Autodesk Inventor part; units mm, degrees
ref_plane "YZ Plane" through (0, 0, 0) normal (1, 0, 0) x (0, 1, 0)
ref_plane "XZ Plane" through (0, 0, 0) normal (0, 1, 0) x (-1, 0, 0)
ref_plane "XY Plane" through (0, 0, 0) normal (0, 0, 1) x (1, 0, 0)
sketch "Sketch1" plane through (0, 0, 0) normal (1, 0, 0) x (0, 1, 0)
  line L0 (0, 0) -> (40, 0) construction
  line L1 (40, 0) -> (40, 66.5) construction
  line L2 (40, 66.5) -> (0, 66.5) construction
  line L3 (0, 66.5) -> (0, 0) construction
  line L4 (0, 66.5) -> (40, 66.5) construction
  line L5 (40, 66.5) -> (40, 86.5) construction
  line L6 (40, 86.5) -> (0, 86.5)
  line L7 (0, 86.5) -> (0, 66.5) construction
  line L8 (0, 0) -> (40, 0) construction
  line L9 (40, 0) -> (40, -20) construction
  line L10 (40, -20) -> (0, -20) construction
  line L11 (0, -20) -> (0, 0) construction
  line L12 (48.2, 61.45) -> (-8.2, 61.45) construction
  line L13 (-8.2, 61.45) -> (-8.2, 5.05) construction
  line L14 (-8.2, 5.05) -> (48.2, 5.05) construction
  line L15 (48.2, 5.05) -> (48.2, 61.45) construction
  line L16 (48.2, 33.25) -> (-8.2, 33.25) construction
  line L17 (40, 33.25) -> (0, 33.25) construction
  line L18 (43.57, 56.82) -> (-3.57, 56.82) construction
  line L19 (-3.57, 56.82) -> (-3.57, 9.68) construction
  line L20 (-3.57, 9.68) -> (43.57, 9.68) construction
  line L21 (43.57, 9.68) -> (43.57, 56.82) construction
  line L22 (43.57, 56.82) -> (48.2, 56.82) construction
  line L23 (43.57, 56.82) -> (43.57, 61.45) construction
  line L24 (-3.57, 9.68) -> (-8.2, 9.68) construction
  line L25 (-3.57, 9.68) -> (-3.57, 5.05) construction
  line L26 (40, -10) -> (0, -10) construction
  line L27 (40, 76.5) -> (0, 76.5) construction
  circle A0 centre (30, 76.5) radius 2.1
  circle A1 centre (10, 76.5) radius 2.1
  circle A2 centre (30, -10) radius 2.1
  circle A3 centre (10, -10) radius 2.1
  circle A4 centre (43.57, 56.82) radius 2.6 construction
  circle A5 centre (43.57, 9.68) radius 2.6 construction
  circle A6 centre (-3.57, 9.68) radius 2.6 construction
  circle A7 centre (-3.57, 56.82) radius 2.6 construction
  circle A8 centre (-25, 18.25) radius 11.08 construction
  circle A9 centre (-25, 18.25) radius 13 construction
  circle A10 centre (-25, 18.25) radius 2.5
  line L28 (-60, 153.25) -> (-60, -86.75) construction
  circle A11 centre (-60, -86.75) radius 2.6
  circle A12 centre (-60, 153.25) radius 2.6
  line L29 (-120.2, 153.25) -> (-120.2, -86.75) construction
  circle A13 centre (-120.2, -86.75) radius 2.6
  circle A14 centre (-120.2, 153.25) radius 2.6
  circle A15 centre (-60, -86.75) radius 12 construction
  circle A16 centre (-120.2, -86.75) radius 12 construction
  circle A17 centre (-120.2, 153.25) radius 12 construction
  circle A18 centre (-60, 153.25) radius 12 construction
  line L30 (-110, 482.7599) -> (-70, 482.7599) construction
  line L31 (-70, -517.2401) -> (-110, -517.2401) construction
  circle A19 centre (-25, 48.25) radius 2.5
  circle A20 centre (-25, 48.25) radius 11.08 construction
  circle A21 centre (-25, 48.25) radius 13 construction
  circle A22 centre (20, 33.25) radius 11.08 construction
  circle A23 centre (20, 33.25) radius 13 construction
  line L32 (-23.1873, 29.1807) -> (18.1873, 22.3193) construction
  line L33 (18.1873, 44.1807) -> (-23.1873, 37.3193) construction
  line L34 (-120.8333, -99.25) -> (-47.8333, -99.25)
  line L35 (-47.8333, 165.75) -> (-120.8333, 165.75)
  line L36 (-132.8333, 153.75) -> (-132.8333, -87.25)
  line L37 (-60, 153.25) -> (-120.2, 153.25) construction
  line L38 (-120.2, -86.75) -> (-60, -86.75) construction
  line L39 (-60, 153.25) -> (-60, 165.75) construction
  line L40 (-120.2, -86.75) -> (-120.2, -99.25) construction
  line L41 (48.3276, -20) -> (48.3276, 86.5)
  line L42 (17.6122, 86.5) -> (40, 86.5) construction
  arc A24 (-120.8333, 165.75) -> (-132.8333, 153.75) centre (-120.8333, 153.75) ccw
  arc A25 (-132.8333, -87.25) -> (-120.8333, -99.25) centre (-120.8333, -87.25) ccw
  line L43 (48.3276, -20) -> (-47.8333, -99.25)
  line L44 (-47.8333, 165.75) -> (-47.8333, -99.25) construction
  line L45 (-120.2, -86.75) -> (-132.8333, -86.75) construction
  line L46 (-60, 153.25) -> (-47.8333, 153.25) construction
  line L47 (-36.08, 48.25) -> (-36.08, 286.613) construction
  line L48 (-47.8333, 145.75) -> (-47.8333, 86.5)
  line L49 (-47.8333, 86.5) -> (16.8804, 86.5)
  line L50 (-47.8333, -73.3332) -> (16.8804, -20)
  line L51 (-47.8333, -20) -> (16.8804, -20)
  line L52 (-47.8333, -73.3332) -> (-47.8333, -20)
  line L53 (48.3276, 86.5) -> (48.3276, 165.75)
  line L54 (48.3276, 165.75) -> (-47.8333, 165.75)
  line L55 (-47.8333, 145.75) -> (28.3276, 145.75)
  line L56 (28.3276, 145.75) -> (28.3276, 86.5)
  line L57 (-47.8333, 145.75) -> (28.3276, 86.5) construction
  line L58 (-39.6904, 145.75) -> (28.3276, 92.8349)
  line L59 (-47.8333, 139.4151) -> (20.1847, 86.5)
  circle A26 centre (20, 33.25) radius 3.5
  line L60 (20, 33.25) -> (20, 13.25) construction
  line L61 (20, 33.25) -> (20, 53.25) construction
  circle A27 centre (20, 13.25) radius 2.6
  circle A28 centre (20, 53.25) radius 2.6
  point P0 (-132.8333, -99.25)
  point P1 (-132.8333, 165.75)
  point P2 (-47.8333, 139.8332)
  point P3 (0, 86.5)
  point P4 (0, 86.5)
  dimension "d181" = 22.16
  dimension "d156" = 40
  dimension "d157" = 66.5
  dimension "d158" = 40
  dimension "d159" = 20
  dimension "d160" = 40
  dimension "d161" = 20
  dimension "d162" = 56.4
  dimension "d163" = 56.4
  dimension "d164" = 0
  dimension "d165" = 8.2
  dimension "d166" = 47.14
  dimension "d167" = 47.14
  dimension "d168" = 4.2
  dimension "d169" = 20
  dimension "d170" = 10
  dimension "d171" = 10
  dimension "d172" = 20
  dimension "d173" = 4.2
  dimension "d174" = 4.2
  dimension "d175" = 4.2
  dimension "d176" = 5.2
  dimension "d177" = 5.2
  dimension "d178" = 5.2
  dimension "d179" = 5.2
  dimension "d182" = 26
  dimension "d183" = 5
  dimension "d184" = 240
  dimension "d185" = 60
  dimension "d186" = 5.2
  dimension "d187" = 5.2
  dimension "d188" = 5.2
  dimension "d189" = 5.2
  dimension "d190" = 60.2
  dimension "d191" = 24
  dimension "d192" = 24
  dimension "d193" = 24
  dimension "d194" = 24
  dimension "d195" = 40
  dimension "d196" = 1000
  dimension "d198" = 5
  dimension "d199" = 22.16
  dimension "d200" = 26
  dimension "d202" = 22.16
  dimension "d203" = 26
  dimension "d205" = 15
  dimension "d206" = 265
  dimension "d207" = 85
  dimension "d208" = 106.5
  dimension "d209" = 12
  dimension "d210" = 72.8333
  dimension "d212" = 53.25
  dimension "d213" = 85
  dimension "d214" = 132.5
  dimension "d215" = 60.2
  dimension "d216" = 20
  dimension "d217" = 20
  dimension "d218" = 5
  dimension "d219" = 5
  dimension "d220" = 7
  dimension "d221" = 20
  dimension "d222" = 20
  dimension "d223" = 5.2
  dimension "d224" = 5.2
extrude "Extrusion1" add sketch "Sketch1" along normal blind 3.175 contours L6 L59 L48 L55 L58 L56 | A25 L36 A24 L35 L54 L53 L41 L43 L34
sketch "Sketch4" plane through (3.175, 0, 0) normal (1, 0, 0) x (0, 0, -1)
  line L0 (20, 16.8804) -> (73.3332, -47.8333)
  line L1 (39.0796, -6.2705) -> (54.5136, 6.4492) construction
  line L2 (99.25, -47.8333) -> (20, 48.3276) construction
  line L3 (46.7966, 0.0893) -> (37.2568, 11.6648) construction
  line L4 (46.7966, 0.0893) -> (56.3364, -11.4861) construction
  circle A0 centre (37.2568, 11.6648) radius 2.6
  circle A1 centre (56.3364, -11.4861) radius 2.6
  line L5 (-145.75, 28.3276) -> (-92.8349, 28.3276)
  line L6 (-119.2924, 28.3276) -> (-119.2924, 48.3276) construction
  line L7 (20, 48.3276) -> (-165.75, 48.3276) construction
  line L8 (-119.2924, 38.3276) -> (-104.2924, 38.3276) construction
  line L9 (-119.2924, 38.3276) -> (-134.2924, 38.3276) construction
  circle A2 centre (-134.2924, 38.3276) radius 2.6
  circle A3 centre (-104.2924, 38.3276) radius 2.6
  point P0 (0, 0)
  point P1 (0, 0)
  dimension "d228" = 30
  dimension "d229" = 15
  dimension "d230" = 15
  dimension "d231" = 5.2
  dimension "d232" = 5.2
  dimension "d233" = 15
  dimension "d234" = 15
  dimension "d235" = 5.2
  dimension "d236" = 5.2
  dimension "d237" = 52.9151
  dimension "d238" = 26.4576
extrude "Extrusion4" cut sketch "Sketch4" against normal through all
fillet "Fillet2" radius 3.175 11 edges at (1.5875, 28.3276, 92.8349) (1.5875, 20.1847, 86.5) (1.5875, -39.6904, 145.75) (1.5875, -47.8333, 139.4151) (1.5875, 16.8804, -20) (1.5875, 48.3276, -20) (1.5875, -47.8333, -20) (1.5875, -47.8333, -73.3332) (1.5875, -47.8333, -99.25) (1.5875, -47.8333, 86.5) (1.5875, 28.3276, 145.75)
chamfer "Chamfer1" distance 10 angle 45 1 edges at (1.5875, 48.3276, 165.75)
sketch "Sketch5" plane through (3.175, 0, 0) normal (1, 0, 0) x (0, 0, -1)
  line L0 (-145.75, -30.4384) -> (-145.75, 25.1526)
  line L1 (-165.75, 38.3276) -> (-165.75, -120.8333)
  line L2 (-145.75, 28.3276) -> (-165.75, 28.3276)
  line L3 (-165.75, 28.3276) -> (-165.75, -21.6724)
  line L4 (-165.75, -21.6724) -> (-145.75, -21.6724)
  line L5 (-145.75, -21.6724) -> (-145.75, 28.3276)
  line L6 (18.5023, 48.3276) -> (-155.75, 48.3276)
  line L7 (-142.575, 28.3276) -> (-99.3275, 28.3276)
  line L8 (-155.75, 28.3276) -> (-155.75, -21.6724) construction
  circle A0 centre (-155.75, 15.8276) radius 2.6
  circle A1 centre (-155.75, -9.1724) radius 2.6
  point P0 (0, 0)
  dimension "d239" = 50
  dimension "d241" = 5.2
  dimension "d242" = 5.2
  dimension "d243" = 12.5
  dimension "d244" = 12.5
extrude "Extrusion5" cut sketch "Sketch5" against normal up to next contours A0 | A1
properties part number "X Axis V Wheel Frame Machined"
Verification items for the finished model (mm, model axes). A direction names the side the tool comes from. Give positions to 0.01 mm unless a question says otherwise; leave off trailing zeros. Loops run counter-clockwise (first coordinate to the right, second up) from the corner with the lowest first, then second, coordinate; pieces in that order, holes last.
1. Section check A-A, the plane z = 33.25. Enter the section's corners in (x, y) (3 decimals).
2. Thickness scan on line 1 (Z direction, x = 0.75, y = -60); line 2 (Z direction, x = 0.35, y = -122.5); line 3 (Z direction, x = 1.2, y = -21.5). Record the ranges inside material, lowest first.
3. Go/stop test with a flat-tipped pin: pin 1 Ø1.6 at (x, y) = (1.5, -15.5) entering from -Z. Record where the tip stops, or that it passes through.
4. Section check C-C, the plane x = 2.15. Count the separate pieces of the cut face and the enclosed holes in it, then the cut area to 3 significant figures.
5. Set-up check for faces 5 (the flat face through (1.565, -15.302, 114.107)), 6 (the cylindrical face through (1.565, -129.411, 162.141)): record each of +Z, -Z, +X, -X, +Y, -Y from which the full face is reachable in a straight line by a thin tool's end or side.
6. Mould release check, pull along Y, two halves, no side actions. Record for faces 1 (the flat face through (3.175, -44, 35)), 2 (the cylindrical face through (1.565, -62.063, 154.832)), 3 (the flat face through (1.57, -16.66, -47.64)), 4 (the flat face through (1.565, 0.768, -59.196)): released by +Y, released by -Y, zero draft, split by the parting line, or undercut.
7. Section check B-B, the plane y = -60. Enter the section's corners in (x, z) (3 decimals), then the cut area to 3 significant figures.
Geometry says:
1. outline: (0, -132.833) - (3.175, -132.833) - (3.175, 16.5) - (0, 16.5) - close; (0, 23.5) - (3.175, 23.5) - (3.175, 48.328) - (0, 48.328) - close
2. line 1: z = -99.25 to -89.35, -84.15 to 150.65, 155.85 to 165.75
2. line 2: z = -99.13 to -87.96, -85.54 to 152.04, 154.46 to 165.63
2. line 3: z = -77.55 to -51.63, -20 to 86.5, 118.93 to 131.6, 145.75 to 165.75
3. pin 1: stops at z = -73.26
4. separate pieces: 1
4. enclosed holes: 22
4. area: 38,500 mm2
5. face 5: +X, -X
5. face 6: +Z, +X, -X, -Y
6. face 1: zero draft
6. face 2: undercut
6. face 3: undercut
6. face 4: released by +Y
7. outline: (0, -99.25) - (3.175, -99.25) - (3.175, -89.35) - (0, -89.35) - close; (0, -84.15) - (3.175, -84.15) - (3.175, 150.65) - (0, 150.65) - close; (0, 155.85) - (3.175, 155.85) - (3.175, 165.75) - (0, 165.75) - close
7. area: 808 mm2
